Verification items for the finished model (mm, model axes). Round coordinates to 2 decimals unless told otherwise and drop trailing zeros. Answer in a Markdown table with one row per item. Add a question column.
1. Material ranges on probe 1 along X at (y, z) = (2.9, 51.5); probe 2 along X at (y, z) = (1.95, 14); probe 3 along X at (y, z) = (1.85, 42), recorded low to high.
2. Sectioned sample at A-A on y = 1.5. Count the separate pieces of the cut face and the enclosed holes in it, plus the area to 3 significant figures.
3. Go/stop test with flat-tipped pins: pin 1 Ø1 at (x, y) = (7, 2.5) entering from -Z; pin 2 Ø1 at (x, y) = (24, 2) entering from +Z; pin 3 Ø1 at (x, y) = (23, 1) entering from -Z. Record where each tip stops, or that it passes through.
```python
from build123d import *

# Parameters (mm, degrees)
MODEL_R             = 76.199999999
MODEL_R_2           = 1.5875
BOSS_EXTRUDE1_DEPTH = 3.175


with BuildPart() as part:
    # Model → Boss-Extrude1 (new body)
    with BuildSketch(Plane(origin=(0, 0, 0), x_dir=(1, 0, 0), z_dir=(0, 1, 0))):
        with Locations(Location((1e-09, -4e-09, 0), (0, 0, 270))):
            Circle(MODEL_R)
        with Locations(Location((-21.062340001, 37.48772538, 0), (0, 0, 270))):
            Circle(MODEL_R_2, mode=Mode.SUBTRACT)
        with Locations(Location((24.022659999, -28.55227462, 0), (0, 0, 270))):
            Circle(MODEL_R_2, mode=Mode.SUBTRACT)
        with Locations(Location((-34.925, -60.491874454, 0), (0, 0, 270))):
            Circle(MODEL_R_2, mode=Mode.SUBTRACT)
        with Locations(Location((-60.491874454, -34.925, 0), (0, 0, 270))):
            Circle(MODEL_R_2, mode=Mode.SUBTRACT)
        with Locations(Location((-69.85, 0, 0), (0, 0, 270))):
            Circle(MODEL_R_2, mode=Mode.SUBTRACT)
        with Locations(Location((-60.491874454, 34.925, 0), (0, 0, 270))):
            Circle(MODEL_R_2, mode=Mode.SUBTRACT)
        with Locations(Location((0, 69.85, 0), (0, 0, 270))):
            Circle(MODEL_R_2, mode=Mode.SUBTRACT)
        with Locations(Location((34.925, 60.491874454, 0), (0, 0, 270))):
            Circle(MODEL_R_2, mode=Mode.SUBTRACT)
        with Locations(Location((60.491874454, 34.925, 0), (0, 0, 270))):
            Circle(MODEL_R_2, mode=Mode.SUBTRACT)
        with Locations(Location((69.85, 0, 0), (0, 0, 270))):
            Circle(MODEL_R_2, mode=Mode.SUBTRACT)
        with Locations(Location((60.491874454, -34.925, 0), (0, 0, 270))):
            Circle(MODEL_R_2, mode=Mode.SUBTRACT)
        with Locations(Location((34.925, -60.491874454, 0), (0, 0, 270))):
            Circle(MODEL_R_2, mode=Mode.SUBTRACT)
        with Locations(Location((-24.237340001, -28.55227462, 0), (0, 0, 270))):
            Circle(MODEL_R_2, mode=Mode.SUBTRACT)
        with Locations(Location((0, -69.85, 0), (0, 0, 270))):
            Circle(MODEL_R_2, mode=Mode.SUBTRACT)
        with Locations(Location((18.0785103, -67.469918966, 0), (0, 0, 270))):
            Circle(MODEL_R_2, mode=Mode.SUBTRACT)
        with Locations(Location((49.391408667, -49.391408667, 0), (0, 0, 270))):
            Circle(MODEL_R_2, mode=Mode.SUBTRACT)
        with Locations(Location((67.469918966, -18.0785103, 0), (0, 0, 270))):
            Circle(MODEL_R_2, mode=Mode.SUBTRACT)
        with Locations(Location((67.469918966, 18.0785103, 0), (0, 0, 270))):
            Circle(MODEL_R_2, mode=Mode.SUBTRACT)
        with Locations(Location((49.391408667, 49.391408667, 0), (0, 0, 270))):
            Circle(MODEL_R_2, mode=Mode.SUBTRACT)
        with Locations(Location((18.0785103, 67.469918966, 0), (0, 0, 270))):
            Circle(MODEL_R_2, mode=Mode.SUBTRACT)
        with Locations(Location((-18.0785103, 67.469918966, 0), (0, 0, 270))):
            Circle(MODEL_R_2, mode=Mode.SUBTRACT)
        with Locations(Location((-49.391408667, 49.391408667, 0), (0, 0, 270))):
            Circle(MODEL_R_2, mode=Mode.SUBTRACT)
        with Locations(Location((-67.469918966, 18.0785103, 0), (0, 0, 270))):
            Circle(MODEL_R_2, mode=Mode.SUBTRACT)
        with Locations(Location((-67.469918966, -18.0785103, 0), (0, 0, 270))):
            Circle(MODEL_R_2, mode=Mode.SUBTRACT)
        with Locations(Location((-49.391408667, -49.391408667, 0), (0, 0, 270))):
            Circle(MODEL_R_2, mode=Mode.SUBTRACT)
        with Locations(Location((-18.0785103, -67.469918966, 0), (0, 0, 270))):
            Circle(MODEL_R_2, mode=Mode.SUBTRACT)
        with Locations(Location((20.847659999, 37.48772538, 0), (0, 0, 270))):
            Circle(MODEL_R_2, mode=Mode.SUBTRACT)
        with Locations(Location((-34.925, 60.491874454, 0), (0, 0, 270))):
            Circle(MODEL_R_2, mode=Mode.SUBTRACT)
        with BuildLine():
            Line((-39.894076643, -8.73125), (-52.709304986, -30.927876602))
            ThreePointArc((-52.709304986, -30.927876602), (-54.096237861, -31.721580355), (-55.470892632, -30.906796514))
            ThreePointArc((-55.470892632, -30.906796514), (-60.307423447, -19.881264479), (-62.975977178, -8.141025641))
            ThreePointArc((-62.975977178, -8.141025641), (-62.593897589, -6.889392349), (-61.401577748, -6.35))
            Line((-61.401577748, -6.35), (-41.268891971, -6.35))
            ThreePointArc((-41.268891971, -6.35), (-39.894076643, -7.14375), (-39.894076643, -8.73125))
        make_face(mode=Mode.SUBTRACT)
        with BuildLine():
            Line((39.894076642, 8.731249996), (52.709304986, 30.927876598))
            ThreePointArc((52.709304986, 30.927876598), (54.09623786, 31.721580351), (55.470892632, 30.906796511))
            ThreePointArc((55.470892632, 30.906796511), (60.307423447, 19.881264475), (62.975977179, 8.141025637))
            ThreePointArc((62.975977179, 8.141025637), (62.593897589, 6.889392344), (61.401577747, 6.349999996))
            Line((61.401577747, 6.349999996), (41.26889197, 6.349999996))
            ThreePointArc((41.26889197, 6.349999996), (39.894076642, 7.143749997), (39.894076642, 8.731249996))
        make_face(mode=Mode.SUBTRACT)
        with BuildLine():
            Line((-35.982315329, 14.655880652), (-49.529418969, 38.120152452))
            ThreePointArc((-49.529418969, 38.120152452), (-49.737272965, 39.037652431), (-49.389337066, 39.911694823))
            ThreePointArc((-49.389337066, 39.911694823), (-42.917583758, 46.800972253), (-35.494871794, 52.653243734))
            ThreePointArc((-35.494871794, 52.653243734), (-33.862029167, 52.738493705), (-33.020000001, 51.336912639))
            Line((-33.020000001, 51.336912639), (-33.020000001, 15.449630652))
            ThreePointArc((-33.020000001, 15.449630652), (-34.196624767, 13.916223405), (-35.982315329, 14.655880652))
        make_face(mode=Mode.SUBTRACT)
        with BuildLine():
            Line((41.268891969, -6.350000005), (61.401577747, -6.350000005))
            ThreePointArc((61.401577747, -6.350000005), (62.593897589, -6.889392353), (62.975977179, -8.141025645))
            ThreePointArc((62.975977179, -8.141025645), (60.307423447, -19.881264484), (55.470892631, -30.906796519))
            ThreePointArc((55.470892631, -30.906796519), (54.09623786, -31.72158036), (52.709304985, -30.927876606))
            Line((52.709304985, -30.927876606), (39.894076642, -8.731250005))
            ThreePointArc((39.894076642, -8.731250005), (39.894076642, -7.143750005), (41.268891969, -6.350000005))
        make_face(mode=Mode.SUBTRACT)
        with BuildLine():
            Line((17.145000001, 39.997748357), (17.143275501, 35.271178328))
            ThreePointArc((17.143275501, 35.271178328), (17.606151348, 34.14483939), (18.730764569, 33.677786336))
            Line((18.730764569, 33.677786336), (26.5373616, 33.677786336))
            Line((26.5373616, 33.677786336), (26.5373616, -24.742213664))
            Line((26.5373616, -24.742213664), (23.042500002, -24.742213664))
            ThreePointArc((23.042500002, -24.742213664), (21.919967987, -25.207181649), (21.455000002, -26.329713664))
            Line((21.455000002, -26.329713664), (21.455000002, -29.667200004))
            ThreePointArc((21.455000002, -29.667200004), (21.919967987, -30.789732019), (23.042500002, -31.254700004))
            Line((23.042500002, -31.254700004), (25.082500001, -31.254700004))
            ThreePointArc((25.082500001, -31.254700004), (26.205032016, -31.719667989), (26.670000001, -32.842200004))
            Line((26.670000001, -32.842200004), (26.670000001, -44.767500004))
            ThreePointArc((26.670000001, -44.767500004), (26.205032016, -45.890032019), (25.082500001, -46.355000004))
            Line((25.082500001, -46.355000004), (21.907500001, -46.355000004))
            ThreePointArc((21.907500001, -46.355000004), (20.784967986, -46.819967989), (20.320000001, -47.942500004))
            Line((20.320000001, -47.942500004), (20.320000001, -59.010601594))
            ThreePointArc((20.320000001, -59.010601594), (20.013645009, -59.948057576), (19.212820514, -60.523693943))
            ThreePointArc((19.212820514, -60.523693943), (1e-09, -63.500000004), (-19.212820512, -60.523693943))
            ThreePointArc((-19.212820512, -60.523693943), (-20.013645007, -59.948057576), (-20.319999999, -59.010601594))
            Line((-20.319999999, -59.010601594), (-20.319999999, -47.942500004))
            ThreePointArc((-20.319999999, -47.942500004), (-20.784967984, -46.819967989), (-21.907499999, -46.355000004))
            Line((-21.907499999, -46.355000004), (-25.082499999, -46.355000004))
            ThreePointArc((-25.082499999, -46.355000004), (-26.205032014, -45.890032019), (-26.669999999, -44.767500004))
            Line((-26.669999999, -44.767500004), (-26.669999999, -32.842200004))
            ThreePointArc((-26.669999999, -32.842200004), (-26.205032014, -31.719667989), (-25.082499999, -31.254700004))
            Line((-25.082499999, -31.254700004), (-23.0425, -31.254700004))
            ThreePointArc((-23.0425, -31.254700004), (-21.919967985, -30.789732019), (-21.455, -29.667200004))
            Line((-21.455, -29.667200004), (-21.455, -26.329713664))
            ThreePointArc((-21.455, -26.329713664), (-21.919967985, -25.207181649), (-23.0425, -24.742213664))
            Line((-23.0425, -24.742213664), (-26.7518384, -24.742213664))
            Line((-26.7518384, -24.742213664), (-26.7518384, 33.677786336))
            Line((-26.7518384, 33.677786336), (-18.732499999, 33.677786336))
            ThreePointArc((-18.732499999, 33.677786336), (-17.609967984, 34.142754321), (-17.144999999, 35.265286336))
            Line((-17.144999999, 35.265286336), (-17.144999999, 39.997748357))
            ThreePointArc((-17.144999999, 39.997748357), (-17.609967984, 41.120280372), (-18.732499999, 41.585248357))
            ThreePointArc((-18.732499999, 41.585248357), (-19.855032014, 42.050216341), (-20.319999999, 43.172748357))
            Line((-20.319999999, 43.172748357), (-20.319999999, 59.010601586))
            ThreePointArc((-20.319999999, 59.010601586), (-20.013645007, 59.948057567), (-19.212820512, 60.523693934))
            ThreePointArc((-19.212820512, 60.523693934), (1e-09, 63.499999996), (19.212820514, 60.523693934))
            ThreePointArc((19.212820514, 60.523693934), (20.013645009, 59.948057567), (20.320000001, 59.010601586))
            Line((20.320000001, 59.010601586), (20.320000001, 43.172748357))
            ThreePointArc((20.320000001, 43.172748357), (19.855032016, 42.050216342), (18.732500001, 41.585248357))
            ThreePointArc((18.732500001, 41.585248357), (17.609967986, 41.120280372), (17.145000001, 39.997748357))
        make_face(mode=Mode.SUBTRACT)
        with BuildLine():
            Line((33.020000001, 15.449630654), (33.020000001, 51.336912641))
            ThreePointArc((33.020000001, 51.336912641), (33.862029168, 52.738493708), (35.494871796, 52.653243734))
            ThreePointArc((35.494871796, 52.653243734), (42.91758376, 46.800972253), (49.389337068, 39.911694824))
            ThreePointArc((49.389337068, 39.911694824), (49.737272966, 39.037652431), (49.529418969, 38.120152454))
            Line((49.529418969, 38.120152454), (35.982315329, 14.655880654))
            ThreePointArc((35.982315329, 14.655880654), (34.196624767, 13.916223406), (33.020000001, 15.449630654))
        make_face(mode=Mode.SUBTRACT)
        with BuildLine():
            Line((35.982315328, -14.655880662), (49.529418968, -38.120152462))
            ThreePointArc((49.529418968, -38.120152462), (49.737272966, -39.037652439), (49.389337068, -39.911694832))
            ThreePointArc((49.389337068, -39.911694832), (42.91758376, -46.800972262), (35.494871795, -52.653243743))
            ThreePointArc((35.494871795, -52.653243743), (33.862029167, -52.738493716), (33.020000001, -51.336912649))
            Line((33.020000001, -51.336912649), (33.020000001, -15.449630662))
            ThreePointArc((33.020000001, -15.449630662), (34.196624766, -13.916223414), (35.982315328, -14.655880662))
        make_face(mode=Mode.SUBTRACT)
        with BuildLine():
            Line((-49.529418969, -38.120152461), (-35.982315328, -14.65588066))
            ThreePointArc((-35.982315328, -14.65588066), (-34.196624764, -13.91622341), (-33.019999999, -15.449630662))
            Line((-33.019999999, -15.449630662), (-33.019999999, -51.336912649))
            ThreePointArc((-33.019999999, -51.336912649), (-33.862029166, -52.738493716), (-35.494871794, -52.653243743))
            ThreePointArc((-35.494871794, -52.653243743), (-42.917583758, -46.800972262), (-49.389337066, -39.911694832))
            ThreePointArc((-49.389337066, -39.911694832), (-49.737272965, -39.037652439), (-49.529418969, -38.120152461))
        make_face(mode=Mode.SUBTRACT)
        with BuildLine():
            Line((-41.26889197, 6.349999996), (-61.401577748, 6.349999996))
            ThreePointArc((-61.401577748, 6.349999996), (-62.593897588, 6.889392345), (-62.975977177, 8.141025637))
            ThreePointArc((-62.975977177, 8.141025637), (-60.307423445, 19.881264475), (-55.470892629, 30.906796511))
            ThreePointArc((-55.470892629, 30.906796511), (-54.096237858, 31.721580351), (-52.709304983, 30.927876598))
            Line((-52.709304983, 30.927876598), (-39.89407664, 8.731249996))
            ThreePointArc((-39.89407664, 8.731249996), (-39.89407664, 7.143749995), (-41.26889197, 6.349999996))
        make_face(mode=Mode.SUBTRACT)
    extrude(amount=BOSS_EXTRUDE1_DEPTH)


solid = part.part
```
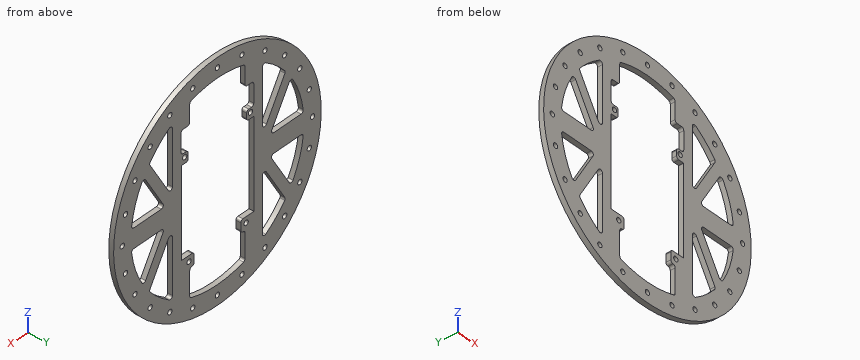
Geometry check:
| question | item | result |
|---|---|---|
| 1 | probe 1 | x = -56.16 to -37.15, -33.03 to -20.32, 20.32 to 33.03, 37.15 to 56.16 |
| 1 | probe 2 | x = -74.9 to -61.94, -42.94 to -35.25, -33.96 to -26.75, 26.54 to 33.96, 35.25 to 42.94, 61.94 to 74.9 |
| 1 | probe 3 | x = -63.58 to -47.63, -33.02 to -26.67, 26.67 to 33.02, 47.63 to 63.58 |
| 2 | separate pieces | 1 |
| 2 | enclosed holes | 37 |
| 2 | area | 9,060 mm2 |
| 3 | pin 1 | stops at z = -75.92 |
| 3 | pin 2 | stops at z = 72.49 |
| 3 | pin 3 | stops at z = -72.8 |
